from build123d import *

# Parameters (mm, degrees)
F0_R     = 60
F0_R_2   = 57.5
F1_DEPTH = 25
F2_R     = 10
F3_DEPTH = 60.001
F5_DEPTH = 60.0010001012
F7_DEPTH = 25.0010001
F8_R     = 5


# Not quite as in the source:
# - a feature names something its author has since deleted; it is built from what else it names


with BuildPart() as f1:
    # F0 (on Top) → F1 (new body)
    with BuildSketch(Plane.XY):
        Circle(F0_R)
        Circle(F0_R_2, mode=Mode.SUBTRACT)
    extrude(amount=F1_DEPTH)

    # F2 (on Front) → F3 (cut, through all)
    with BuildSketch(Plane.XZ):
        Circle(F2_R)
    extrude(amount=-F3_DEPTH, mode=Mode.SUBTRACT)

    # F4 (on Front) → F5 (cut, through all)
    with BuildSketch(Plane.XZ):
        Polygon((-20, 4.6551390551), (-20, 18.0386640131), (-45.0213760883, 18.0386640131), align=None)
        Polygon((45.0213760883, 18.0386640131), (20, 18.0386640131), (20, 4.6551390551), align=None)
    extrude(amount=-F5_DEPTH, mode=Mode.SUBTRACT)

    # F6 (on Top) → F7 (cut, through all)
    with BuildSketch(Plane.XY):
        Polygon((66.0135835631, -64.9920968146), (0, 0), (-63.9864164369, -64.9920968146), align=None)
    extrude(amount=F7_DEPTH, mode=Mode.SUBTRACT)

    # F8
    f8_edges = [f1.edges().sort_by_distance(p)[0] for p in [
        (-41.217352, -41.865169, 25),
        (-41.217352, -41.865169, 0),
        (41.865169, -41.217352, 25),
        (41.865169, -41.217352, 0),
    ]]
    fillet(f8_edges, radius=F8_R)


solid = f1.part
For this review, take the finished solid that the model builds, in its own axes (mm). A direction names the side the tool comes from. Give positions to 0.01 mm unless a question says otherwise; leave off trailing zeros. Loops run counter-clockwise (first coordinate to the right, second up) from the corner with the lowest first, then second, coordinate; pieces in that order, holes last. Notation, with made-up numbers: M -32,40.5 L 12,40.5 A24 ccw 12,62.5 Z; hole C -14.75,10.25 d4. An arc over 180 degrees is marked long. Put each result on its own line as item: value. Start each with the question number.
(1) Add section D-D, the plane x = 0. Write out the cut boundary in (y, z).
(2) Add section A-A, the plane x = -22. Write out the cut boundary in (y, z).
(3) Add section B-B, the plane y = -29.5. Write out the cut boundary in (x, z).
(4) Machinability: for faces 1 (the cylindrical face through (42.856, -40.083, 23.574)), 2 (the cylindrical face through (42.83, -40.06, 1.43)), 3 (the flat face through (-20, 55, 11)), which of the approach directions +Z, -Z, +X, -X, +Y, -Y give a long, thin tool a straight path to every point of the face, cutting with its end or side? Answer none if there is none.
(5) The part is to be moulded in two halves that separate along Z. For faces 4 (the flat face through (55, 18, 0)), 5 (the flat face through (-33.496, 47.66, 11.874)), 6 (the flat face through (-18, 55, 25)), say which applies: +Z half, -Z half, draft (parallel to the pull), parting line (faces both ways), or undercut.
(6) For pin 1 (1.5 mm diameter, centred on y = 5, z = 16.5, fed in from +X); pin 2 (1.3 mm diameter, centred on y = 55.5, z = 11, fed in from -X); pin 3 (5 mm diameter, centred on x = 29.5, z = 7, fed in from -Y); pin 4 (10.5 mm diameter, centred on x = -31, y = 44, fed in from -Z), all flat-tipped, find the tip position at first contact; note any pin that passes through.
(7) Add section C-C, the plane z = 7.75. Write out the cut boundary in (x, y).
(8) Wall thickness on L1, parallel to X at y = 0, z = 5.5; L2, parallel to Y at x = 0, z = 15; L3, parallel to X at y = -8.5, z = 4: over which ranges is each line inside the solid? List them lowest first.
Result:
1. outline: M 57.5,10 L 60,10 L 60,25 L 57.5,25 Z
2. outline: M 53.12,0 L 55.82,0 L 55.82,5.72 L 53.12,5.72 Z; M 53.12,18.04 L 55.82,18.04 L 55.82,25 L 53.12,25 Z
3. outline: M -52.25,0 L -49.36,0 L -49.36,25 L -52.25,25 Z; M 49.36,0 L 52.25,0 L 52.25,25 L 49.36,25 Z
4. face 1: +Z, -Y
4. face 2: -Z, -Y
4. face 3: +Y, -Y
5. face 4: -Z half
5. face 5: undercut
5. face 6: +Z half
6. pin 1: stops at x = 59.85
6. pin 2: stops at x = -20
6. pin 3: stops at y = 47.77
6. pin 4: stops at z = 0
7. outline: M -42.09,-42.76 L -40.34,-40.97 A57.5 cw -25.79,51.39 L -25.79,54.18 A60 ccw Z; M -20,53.91 A57.5 cw -6.32,57.15 L -6.32,59.67 A60 ccw -20,56.57 Z; M 6.32,57.15 A57.5 cw 20,53.91 L 20,56.57 A60 ccw 6.32,59.67 Z; M 25.79,51.39 A57.5 cw 40.97,-40.34 L 42.76,-42.09 A60 ccw 25.79,54.18 Z
8. L1: x = -60 to -57.5, 57.5 to 60
8. L2: y = 57.5 to 60
8. L3: x = -59.39 to -56.87, 56.87 to 59.39
